Design review of the part built by this model. Coordinates are the model's own, in mm. Coordinates: 2 decimals unless noted, no trailing zeros. Loops run counter-clockwise (first coordinate to the right, second up) from the corner with the lowest first, then second, coordinate; pieces in that order, holes last. Notation, with made-up numbers: (21.25, 32) -> (55.25, 32) arc R19 ccw to (55.25, 46) -> close; hole circle Ø7 at (59.25, 79.25). An arc over 180 degrees is marked (long way). One line per item, written item: value. Start each with the question number.
1. Add section C-C on x = 43.5. Write out the cut boundary in (y, z), plus the area to 3 significant figures.
2. For probe 1 along X at (y, z) = (-57, 0.8); probe 2 along Y at (x, z) = (102, 0.65); probe 3 along Z at (x, y) = (-96, -6.5), list the stretches that pass through material, from the lowest coordinate up.
3. Insertion check: pin 1 (0.9 mm diameter, centred on y = -2.5, z = 4, fed in from -X); pin 2 (4 mm diameter, centred on x = -69.5, y = -52, fed in from +Z); pin 3 (1.6 mm diameter, centred on y = -61, z = 3, fed in from -X); pin 4 (2.5 mm diameter, centred on x = 102, y = -57, fed in from -Z). Each pin has a flat end and moves straight along its axis. Give the tip position at first contact, or say it passes through.
4. Add section A-A on z = 3.7. Write out the cut boundary in (x, y), plus the area to 3 significant figures.
5. Add section B-B on y = -49.5. Write out the cut boundary in (x, z).
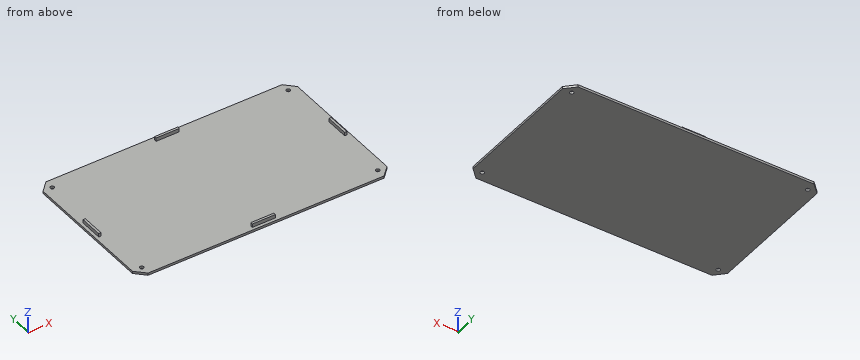
```python
from build123d import *

# Parameters (mm, degrees)
FACETED_REMOVABLE_LID_DEPTH  = 2
SIDE_LOCATOR_1_START         = 2
SKETCH2_W                    = 20
SKETCH2_H                    = 2
SIDE_LOCATOR_1_DEPTH         = 3
END_LOCATOR_1_START          = 2
SKETCH3_W                    = 2
SKETCH3_H                    = 20
END_LOCATOR_1_DEPTH          = 3
SKETCH4_W                    = 20
SKETCH4_H                    = 2
SIDE_LOCATOR_1_2_DEPTH       = 3
SKETCH5_W                    = 2
SKETCH5_H                    = 20
END_LOCATOR_1_2_DEPTH        = 3
M3_LID_CLEARANCE_1_1_START   = -0.1
SKETCH6_R                    = 1.7
M3_LID_CLEARANCE_1_1_DEPTH   = 2.2
SKETCH7_R                    = 1.7
M3_LID_CLEARANCE_1_1_2_DEPTH = 2.2
SKETCH8_R                    = 1.7
M3_LID_CLEARANCE_1_1_3_DEPTH = 2.2
SKETCH9_R                    = 1.7
M3_LID_CLEARANCE_1_1_4_DEPTH = 2.2


with BuildPart() as part:
    # Sketch1 → Faceted_Removable_Lid (new body)
    with BuildSketch(Plane.XY):
        Polygon((-102, -65), (102, -65), (110, -57), (110, 57), (102, 65), (-102, 65), (-110, 57), (-110, -57), align=None)
    extrude(amount=FACETED_REMOVABLE_LID_DEPTH)

    # Sketch2 → Side_Locator_-1 (add)
    with BuildSketch(Plane.XY.offset(SIDE_LOCATOR_1_START)):
        with Locations((0, -61.3)):
            Rectangle(SKETCH2_W, SKETCH2_H)
    extrude(amount=SIDE_LOCATOR_1_DEPTH)

    # Sketch3 → End_Locator_-1 (add)
    with BuildSketch(Plane.XY.offset(END_LOCATOR_1_START)):
        with Locations((-106.3, 0)):
            Rectangle(SKETCH3_W, SKETCH3_H)
    extrude(amount=END_LOCATOR_1_DEPTH)

    # Sketch4 → Side_Locator_1 2 (add)
    with BuildSketch(Plane.XY.offset(SIDE_LOCATOR_1_START)):
        with Locations((0, 61.3)):
            Rectangle(SKETCH4_W, SKETCH4_H)
    extrude(amount=SIDE_LOCATOR_1_2_DEPTH)

    # Sketch5 → End_Locator_1 2 (add)
    with BuildSketch(Plane.XY.offset(END_LOCATOR_1_START)):
        with Locations((106.3, 0)):
            Rectangle(SKETCH5_W, SKETCH5_H)
    extrude(amount=END_LOCATOR_1_2_DEPTH)

    # Sketch6 → M3_Lid_Clearance_-1_-1 (cut)
    with BuildSketch(Plane.XY.offset(M3_LID_CLEARANCE_1_1_START)):
        with Locations((-102, -57)):
            Circle(SKETCH6_R)
    extrude(amount=M3_LID_CLEARANCE_1_1_DEPTH, mode=Mode.SUBTRACT)

    # Sketch7 → M3_Lid_Clearance_-1_1 2 (cut)
    with BuildSketch(Plane.XY.offset(M3_LID_CLEARANCE_1_1_START)):
        with Locations((-102, 57)):
            Circle(SKETCH7_R)
    extrude(amount=M3_LID_CLEARANCE_1_1_2_DEPTH, mode=Mode.SUBTRACT)

    # Sketch8 → M3_Lid_Clearance_1_-1 3 (cut)
    with BuildSketch(Plane.XY.offset(M3_LID_CLEARANCE_1_1_START)):
        with Locations((102, -57)):
            Circle(SKETCH8_R)
    extrude(amount=M3_LID_CLEARANCE_1_1_3_DEPTH, mode=Mode.SUBTRACT)

    # Sketch9 → M3_Lid_Clearance_1_1 4 (cut)
    with BuildSketch(Plane.XY.offset(M3_LID_CLEARANCE_1_1_START)):
        with Locations((102, 57)):
            Circle(SKETCH9_R)
    extrude(amount=M3_LID_CLEARANCE_1_1_4_DEPTH, mode=Mode.SUBTRACT)


solid = part.part
```
Worked answers:
1. outline: (-65, 0) -> (65, 0) -> (65, 2) -> (-65, 2) -> close
1. area: 260 mm²
2. probe 1: x = -110 to -103.7, -100.3 to 100.3, 103.7 to 110
2. probe 2: y = -65 to -58.7, -55.3 to 55.3, 58.7 to 65
2. probe 3: z = 0 to 2
3. pin 1: stops at x = -107.3
3. pin 2: stops at z = 2
3. pin 3: stops at x = -10
3. pin 4: passes through
4. outline: (-107.3, -10) -> (-105.3, -10) -> (-105.3, 10) -> (-107.3, 10) -> close; (-10, -62.3) -> (10, -62.3) -> (10, -60.3) -> (-10, -60.3) -> close; (-10, 60.3) -> (10, 60.3) -> (10, 62.3) -> (-10, 62.3) -> close; (105.3, -10) -> (107.3, -10) -> (107.3, 10) -> (105.3, 10) -> close
4. area: 160 mm²
5. outline: (-110, 0) -> (110, 0) -> (110, 2) -> (-110, 2) -> close
